Verification items for the finished model (mm, model axes). Give positions to 0.01 mm unless a question says otherwise; leave off trailing zeros. Write each loop counter-clockwise with the first axis right and the second up, starting at its lowest first coordinate (ties: lowest second). Pieces come first, ordered by that corner, then holes. Notation, with made-up numbers: (85.25, 59.5) -> (122.25, 59.5) arc R14 ccw to (122.25, 64.5) -> close; hole circle Ø8 at (-20.5, 68.5). An arc over 180 degrees is marked (long way). Answer as CSV lines item,"result". Start each with the question number.
1) Material ranges on L1, parallel to X at y = 1.75, z = -5; L2, parallel to Z at x = 32, y = 1.85; L3, parallel to X at y = 1.6, z = -4.5, recorded low to high.
2) Gauge pin test, flat ends, axial feed: pin 1 Ø1 at (x, y) = (50, 1.5) entering from +Z; pin 2 Ø2.5 at (x, z) = (0, -5) entering from +Y. Record the tip position at first contact, or that the pin passes through.
3) Sectioned sample at D-D on x = 59.5. Record the cut outline in (y, z).
4) Sectioned sample at A-A on x = 29. Record the cut outline in (y, z), and give its area (3 significant figures).
5) Sectioned sample at C-C on z = 12. Record the cut outline in (x, y), and give its area (3 significant figures).
6) Sectioned sample at B-B on y = 2.3. Record the cut outline in (x, z) (3 decimals), and give its area (3 significant figures).
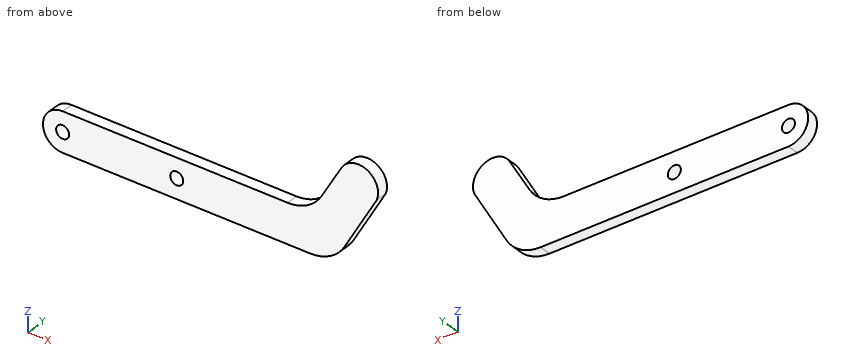
```python
from build123d import *

# Parameters (mm, degrees)
SKETCH_1_R      = 1.65
EXTRUDE_1_DEPTH = 3


with BuildPart() as part:
    # 草图1 → 凸台-拉伸1 (new body)
    with BuildSketch(Plane(origin=(0, 0, 0), x_dir=(1, 0, 0), z_dir=(0, 1, 0))):
        with BuildLine():
            Line((0, 0), (57.2, 0))
            ThreePointArc((57.2, 0), (62.2, -1.339745962), (65.860254038, -5))
            Line((65.860254038, -5), (70.856051038, -13.652974229))
            ThreePointArc((70.856051038, -13.652974229), (77.317543945, -15.675946643), (79.870682341, -9.404998366))
            Line((79.870682341, -9.404998366), (71.687928066, 4.951757862))
            ThreePointArc((71.687928066, 4.951757862), (68.024063165, 8.646316517), (63, 10))
            Line((63, 10), (0, 10))
            ThreePointArc((0, 10), (-5, 5), (0, 0))
        make_face()
        with Locations(Location((0, 5, 0), (0, 0, 270))):
            Circle(SKETCH_1_R, mode=Mode.SUBTRACT)
        with Locations(Location((29, 5, 0), (0, 0, 270))):
            Circle(SKETCH_1_R, mode=Mode.SUBTRACT)
    extrude(amount=EXTRUDE_1_DEPTH)


solid = part.part
```
Ans:
1,L1,"x = -5 to -1.65, 1.65 to 27.35, 30.65 to 71.66"
1,L2,"z = -10 to 0"
1,L3,"x = -4.97 to -1.57, 1.57 to 27.43, 30.57 to 71.95"
2,pin 1,"stops at z = 0"
2,pin 2,"passes through"
3,outline,"(0, -10) -> (3, -10) -> (3, 0.27) -> (0, 0.27) -> close"
4,outline,"(0, -10) -> (3, -10) -> (3, -6.65) -> (0, -6.65) -> close; (0, -3.35) -> (3, -3.35) -> (3, 0) -> (0, 0) -> close"
4,area,"20.1 mm²"
5,outline,"(69.9, 0) -> (80.11, 0) -> (80.11, 3) -> (69.9, 3) -> close"
5,area,"30.6 mm²"
6,outline,"(0, -10) -> (63, -10) arc R10 ccw to (71.688, -4.952) -> (79.871, 9.405) arc R5 ccw to (70.856, 13.653) -> (65.86, 5) arc R10 cw to (57.2, 0) -> (0, 0) arc R5 ccw to start; hole circle Ø3.3 at (0, -5); hole circle Ø3.3 at (29, -5)"
6,area,"906 mm²"
